Source: CAD feature listing. Evaluate the final solid. Frame: model axes, mm. A direction names the side the tool comes from. Round coordinates to 2 decimals unless told otherwise and drop trailing zeros. Write each loop counter-clockwise with the first axis right and the second up, starting at its lowest first coordinate (ties: lowest second). Pieces come first, ordered by that corner, then holes. Notation, with made-up numbers: (47.5, 25) -> (96.5, 25) arc R21 ccw to (96.5, 46) -> close; hole circle Ø9 at (26, -0.75). An arc over 180 degrees is marked (long way). Put each result on its own line as item: value.
```python
from build123d import *

# Parameters (mm, degrees)
F0_W     = 140
F0_H     = 70
F1_DEPTH = 60
F3_DEPTH = 142
F4_W     = 60
F4_H     = 30
F5_DEPTH = 30


with BuildPart() as f1:
    # F0 (on Top) → F1 (new body)
    with BuildSketch(Plane.XY):
        with Locations((-2.236115, 35)):
            Rectangle(F0_W, F0_H)
    extrude(amount=-F1_DEPTH)

    # F2 (on face) → F3 (cut)
    with BuildSketch(Plane.YZ.offset(67.763885)):
        with BuildLine():
            ThreePointArc((17.5, 0), (35, -17.5), (52.5, 0))
            Line((52.5, 0), (17.5, 0))
        make_face()
    extrude(amount=-F3_DEPTH, mode=Mode.SUBTRACT)

    # F4 (on face) → F5 (cut)
    with BuildSketch(Plane.YZ.offset(67.763885)):
        with Locations((40, -45)):
            Rectangle(F4_W, F4_H)
    extrude(amount=-F5_DEPTH, mode=Mode.SUBTRACT)


solid = f1.part
```
Q1. Material intervals for line 1 (Y direction, x = 35.5, z = -5.5); line 2 (Z direction, x = 39.5, y = 56); line 3 (Y direction, x = 54, z = -14), sorted ascending. Write a range as [from, to].
Ans:
line 1: y = [0, 18.39], [51.61, 70]
line 2: z = [-30, 0]
line 3: y = [0, 24.5], [45.5, 70]
Q2. Cut plane B-B on z = -8.5. Output: boundary loops of the cut face in (x, y).
Ans:
outline: (-72.24, 0) -> (67.76, 0) -> (67.76, 19.7) -> (-72.24, 19.7) -> close; (-72.24, 50.3) -> (67.76, 50.3) -> (67.76, 70) -> (-72.24, 70) -> close
Q3. Cut plane A-A on x = -45. Output: boundary loops of the cut face in (y, z), and give its area (3 significant figures).
Ans:
outline: (0, -60) -> (70, -60) -> (70, 0) -> (52.5, 0) arc R17.5 cw to (17.5, 0) -> (0, 0) -> close
area: 3,720 mm^2
Q4. Pin query (flat end, axial travel): pin 1 (8 mm diameter, centred on y = 57.5, z = -50.5, fed in from +X); pin 2 (9 mm diameter, centred on x = 45.5, y = 53, fed in from -Z). Return the tip coordinate at first contact, or that it passes through.
Ans:
pin 1: stops at x = 37.76
pin 2: stops at z = -30
Q5. Draft query along Y for faces 1 (the flat face through (-3, 9, 0)), 2 (the cylindrical face through (-1.256, 34.615, -17.496)), 3 (the flat face through (-3, 70, -30)). Return one class per face: +Y half, -Y half, draft (parallel to the pull), parting line (faces both ways), or undercut.
Ans:
face 1: draft
face 2: undercut
face 3: +Y half
Q6. Reachability of faces 4 (the flat face through (-72.236, 35, -30)), 5 (the flat face through (53, 40, -30)) from +Z, -Z, +X, -X, +Y, -Y: full face, straight path, thin tool, end or side. Return the list, or none.
Ans:
face 4: +Z, -Z, -X, +Y, -Y
face 5: -Z, +X, +Y
Q7. Cut plane C-C on y = 58.5. Output: boundary loops of the cut face in (x, z), and give its area (3 significant figures).
Ans:
outline: (-72.24, -60) -> (37.76, -60) -> (37.76, -30) -> (67.76, -30) -> (67.76, 0) -> (-72.24, 0) -> close
area: 7,500 mm^2
